Check sheet for the modelled part. Datum: model origin and axes. Units: mm. A direction names the side the tool comes from. Coordinates: 2 decimals unless noted, no trailing zeros. Loops run counter-clockwise (first coordinate to the right, second up) from the corner with the lowest first, then second, coordinate; pieces in that order, holes last. Notation, with made-up numbers: (72.5, 24.5) -> (119.5, 24.5) arc R10 cw to (119.5, 34.5) -> close; hole circle Ø9 at (-13, 85). An arc over 180 degrees is marked (long way). Use one line per item in the form item = value.
from build123d import *

# Parameters (mm, degrees)
ESBO_O1_W                 = 6.35
ESBO_O1_H                 = 48
RESSALTO_EXTRUS_O1_DEPTH  = 15
FURO_ROSCADO_DE_M31_D     = 2.5
FURO_ROSCADO_DE_M31_DEPTH = 10
FURO_ROSCADO_DE_M31_TIP   = 0.751075774
FURO_ROSCADO_DE_M32_D     = 2.5
FURO_ROSCADO_DE_M32_DEPTH = 10
FURO_ROSCADO_DE_M32_TIP   = 0.751075774
FURO_ROSCADO_DE_M33_D     = 2.5
FURO_ROSCADO_DE_M33_DEPTH = 10
FURO_ROSCADO_DE_M33_TIP   = 0.751075774


with BuildPart() as part:
    # Esboço1 → Ressalto-extrusão1 (new body)
    with BuildSketch(Plane.XY):
        with Locations((3.175, 24)):
            Rectangle(ESBO_O1_W, ESBO_O1_H)
    extrude(amount=RESSALTO_EXTRUS_O1_DEPTH)

    # Furo roscado de M31
    with Locations(Plane(origin=(3.175, 0, 11), x_dir=(0, 0, -1), z_dir=(0, -1, 0))):
        with Locations((0, 0), (7, 0)):
            Hole(FURO_ROSCADO_DE_M31_D / 2, depth=FURO_ROSCADO_DE_M31_DEPTH)
            with Locations((0, 0, -(FURO_ROSCADO_DE_M31_DEPTH + FURO_ROSCADO_DE_M31_TIP / 2))):  # 118° drill point
                Cone(0, FURO_ROSCADO_DE_M31_D / 2, FURO_ROSCADO_DE_M31_TIP, mode=Mode.SUBTRACT)

    # Furo roscado de M32
    with Locations(Plane(origin=(3.175, 48, 4), x_dir=(0, 0, 1), z_dir=(0, 1, 0))):
        with Locations((0, 0), (7, 0)):
            Hole(FURO_ROSCADO_DE_M32_D / 2, depth=FURO_ROSCADO_DE_M32_DEPTH)
            with Locations((0, 0, -(FURO_ROSCADO_DE_M32_DEPTH + FURO_ROSCADO_DE_M32_TIP / 2))):  # 118° drill point
                Cone(0, FURO_ROSCADO_DE_M32_D / 2, FURO_ROSCADO_DE_M32_TIP, mode=Mode.SUBTRACT)

    # Furo roscado de M33
    with Locations(Plane(origin=(3.175, 34, 15), x_dir=(1, 0, 0), z_dir=(0, 0, 1))):
        with Locations((0, 0)):
            Hole(FURO_ROSCADO_DE_M33_D / 2, depth=FURO_ROSCADO_DE_M33_DEPTH)
            with Locations((0, 0, -(FURO_ROSCADO_DE_M33_DEPTH + FURO_ROSCADO_DE_M33_TIP / 2))):  # 118° drill point
                Cone(0, FURO_ROSCADO_DE_M33_D / 2, FURO_ROSCADO_DE_M33_TIP, mode=Mode.SUBTRACT)


solid = part.part
(1) Section check B-B, the plane y = 3. Record the boundary of the cut face in (x, z) (3 decimals), plus the area to 3 significant figures.
Established:
outline = (0, 0) -> (6.35, 0) -> (6.35, 15) -> (0, 15) -> close; hole circle Ø2.5 at (3.175, 4); hole circle Ø2.5 at (3.175, 11)
area = 85.4 mm²
(2) Scan lines: line 1 along X through (y, z) = (34, 10.5) (3 decimals); line 2 along Y through (x, z) = (3.25, 12.5); line 3 along Z through (x, y) = (4, 6). Record each from-to range of solid material in increasing order.
Established:
line_1 = 0 to 1.925, 4.425 to 6.35
line_2 = 0 to 32.75, 35.25 to 48
line_3 = 0 to 3.06, 4.94 to 10.06, 11.94 to 15
(3) Tool access check on faces 1 (the flat face through (6.35, 24, 7)), 2 (the flat face through (3, 48, 7)), 3 (the cylindrical face through (4.02, 5.07, 10.08)), 4 (the cylindrical face through (3.45, 32.78, 9.93)), 5 (the cylindrical face through (4.414, 42.93, 4.163)). Record the directions out of +Z, -Z, +X, -X, +Y, -Y that give a thin tool (end or side, any length) a straight path to the whole face; none if there is none.
Established:
face_1 = +Z, -Z, +X, +Y, -Y
face_2 = +Z, -Z, +X, -X, +Y
face_3 = -Y
face_4 = +Z
face_5 = +Y
(4) Mould release check, pull along Z, two halves, no side actions. Record for faces 6 (the conical face through (3.292, 34.183, 4.379)), 7 (the flat face through (0, 24, 7)), 8 (the cylindrical face through (4.02, 42.93, 11.92)), 9 (the conical face through (3.32, 10.62, 4.16)): +Z half, -Z half, draft (parallel to the pull), parting line (faces both ways), or undercut.
Established:
face_6 = +Z half
face_7 = draft
face_8 = undercut
face_9 = undercut
(5) Go/stop test with flat-tipped pins: P1, Ø2, axis at x = 3.175, z = 11, coming from the +Y side; P2, Ø2, axis at x = 3.175, z = 4, coming from the -Y side; P3, Ø2, axis at x = 3.175, y = 34, coming from the +Z side. Record where each tip stops, or that it passes through.
Established:
P1 = 37.85
P2 = 10.15
P3 = 4.85
(6) Section check A-A, the plane z = 13.5. Record the boundary of the cut face in (x, y) (3 decimals), plus the area to 3 significant figures.
Established:
outline = (0, 0) -> (6.35, 0) -> (6.35, 48) -> (0, 48) -> close; hole circle Ø2.5 at (3.175, 34)
area = 300 mm²
